Study the drawing (mm; zero at the part's minimum x, y, z) and answer. A direction names the side the tool comes from. Give positions to 0.01 mm unless a question says otherwise; leave off trailing zeros. Write each loop counter-clockwise with the first axis right and the second up, starting at its lowest first coordinate (ties: lowest second). Pieces come first, ordered by that corner, then holes. Notation, with made-up numbers: M 51,82 L 75,82 A11 cw 75,95 Z; hole C -21.5,4 d2. An arc over 180 degrees is marked long. Use a Markdown table: item, result. Add a question column.
Item 1: A cutting plane is placed at D-D on y = 168. Determine the outline of the cut face in (x, z), then the cut area to 3 significant figures.
Item 2: A cutting plane is placed at C-C on y = 114.5. Determine the outline of the cut face in (x, z), then the cut area to 3 significant figures.
Item 3: A cutting plane is placed at A-A on x = 520. Determine the outline of the cut face in (y, z), then the cut area to 3 significant figures.
Item 4: Given P1, Ø4, axis at x = 232.5, y = 174, coming from the +Z side; P2, Ø2, axis at x = 332, z = 324, coming from the +Y side; P3, Ø8, axis at y = 101.5, z = 582.5, coming from the +X side, each flat-ended and moving along its own axis, determine where each tip first touches the part or whether it passes through.
Item 5: For the marked faces 1 and 2, determine the directions among +Z, -Z, +X, -X, +Y, -Y from which every point of the face is accessible in a straight line to the end or side of a thin tool.
Item 6: A cutting plane is placed at B-B on z = 574. Determine the outline of the cut face in (x, y).
Item 7: Consider probe 1 along Y at (x, z) = (338, 386); probe 2 along Z at (x, y) = (143.5, 156); probe 3 along Z at (x, y) = (360, 178). Determine where each line is inside the solid, lowest interval first. Write a range as [from, to].
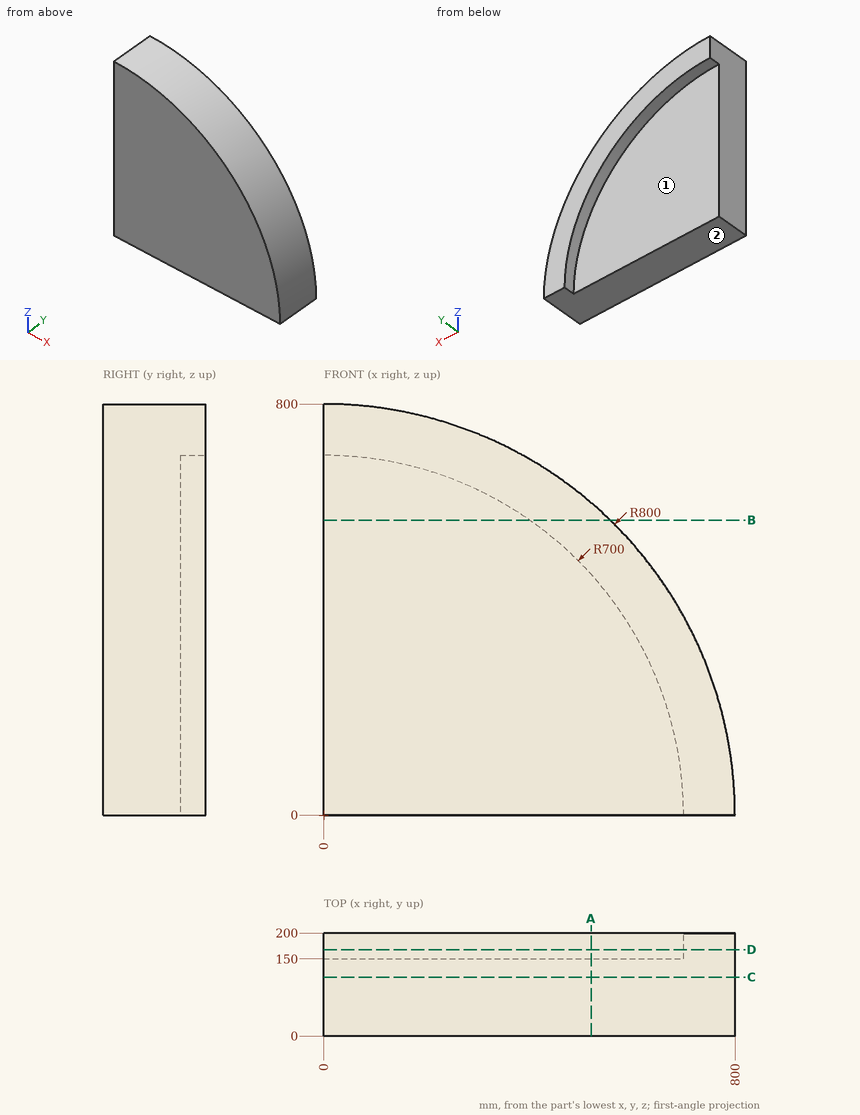
Filled in:
| question | item | result |
|---|---|---|
| 1 | outline | M 0,700 A700 cw 700,0 L 800,0 A800 ccw 0,800 Z |
| 1 | area | 118,000 mm² |
| 2 | outline | M 0,0 L 800,0 A800 ccw 0,800 Z |
| 2 | area | 503,000 mm² |
| 3 | outline | M 0,0 L 150,0 L 150,468.61 L 200,468.61 L 200,607.95 L 0,607.95 Z |
| 3 | area | 98,200 mm² |
| 4 | P1 | z = 766.07 |
| 4 | P2 | y = 150 |
| 4 | P3 | x = 552.57 |
| 5 | face 1 | -Z, -X, +Y |
| 5 | face 2 | -Z, +X, -X, +Y, -Y |
| 6 | outline | M 0,0 L 557.25,0 L 557.25,200 L 400.65,200 L 400.65,150 L 0,150 Z |
| 7 | probe 1 | [0, 150] |
| 7 | probe 2 | [685.13, 787.02] |
| 7 | probe 3 | [600.33, 714.42] |
